Work out the finished part from the listing and answer in its coordinate system (mm). Face numbers are marked on the shaded views. A direction names the side the tool comes from. Give positions to 0.01 mm unless a question says otherwise; leave off trailing zeros. Order: outer loops, then holes, each group sorted by start corner. A loop starts at its lowest first (then second) coordinate and runs counter-clockwise, first axis right, second up. Notation, with made-up numbers: M 37,-22.75 L 82,-22.75 A14 ccw 82,3.25 Z; hole C 53,55 d11. An arc over 180 degrees is marked long. One line per item, written item: value.
from build123d import *

# Parameters (mm, degrees)
BOSS_EXTRUDE1_DEPTH = 66.04
SKETCH2_R           = 2.5
CUT_EXTRUDE1_DEPTH  = 4.175
BOSS_EXTRUDE2_DEPTH = 2.54
SKETCH4_W           = 3.175
SKETCH4_H           = 7.62
CUT_EXTRUDE2_DEPTH  = 25.4
SKETCH5_R           = 1.5
CUT_EXTRUDE3_DEPTH  = 25.4
FILLET1_R           = 3.175


with BuildPart() as part:
    # Sketch1 → Boss-Extrude1 (new body)
    with BuildSketch(Plane.XY):
        Polygon((3.175, -3.175), (15.875, -3.175), (15.875, 0), (0, 0), (0, -15.875), (3.175, -15.875), align=None)
    extrude(amount=-BOSS_EXTRUDE1_DEPTH)

    # Sketch2 → Cut-Extrude1 (cut, through all)
    with BuildSketch(Plane(origin=(3.175, 0, 0), x_dir=(0, 0, -1), z_dir=(1, 0, 0))):
        with Locations((29.95, -9.525)):
            Circle(SKETCH2_R)
        with Locations((9.95, -9.525)):
            Circle(SKETCH2_R)
    extrude(amount=-CUT_EXTRUDE1_DEPTH, mode=Mode.SUBTRACT)

    # Sketch3 → Boss-Extrude2 (add, symmetric)
    with BuildSketch(Plane.XY.offset(-19.685)):
        Polygon((3.175, -15.875), (3.175, -3.175), (15.875, -3.175), align=None)
    extrude(amount=BOSS_EXTRUDE2_DEPTH, both=True)

    # Sketch4 → Cut-Extrude2 (cut)
    with BuildSketch(Plane(origin=(0, 0, -66.04), x_dir=(-1, 0, 0), z_dir=(0, 0, -1))):
        with Locations((-1.5875, -12.065)):
            Rectangle(SKETCH4_W, SKETCH4_H)
    extrude(amount=-CUT_EXTRUDE2_DEPTH, mode=Mode.SUBTRACT)

    # Sketch5 → Cut-Extrude3 (cut)
    with BuildSketch(Plane.XZ.offset(3.175)):
        with Locations((10.375, -34.196688578)):
            Circle(SKETCH5_R)
        with Locations((10.375, -62.196688578)):
            Circle(SKETCH5_R)
    extrude(amount=-CUT_EXTRUDE3_DEPTH, mode=Mode.SUBTRACT)

    # Fillet1
    fillet1_edges = [part.edges().sort_by_distance(p)[0] for p in [
        (15.875, -1.5875, -66.04),
        (1.5875, -15.875, -40.64),
        (1.5875, -8.255, -66.04),
        (1.5875, -15.875, 0),
        (15.875, -1.5875, 0),
    ]]
    fillet(fillet1_edges, radius=FILLET1_R)


solid = part.part
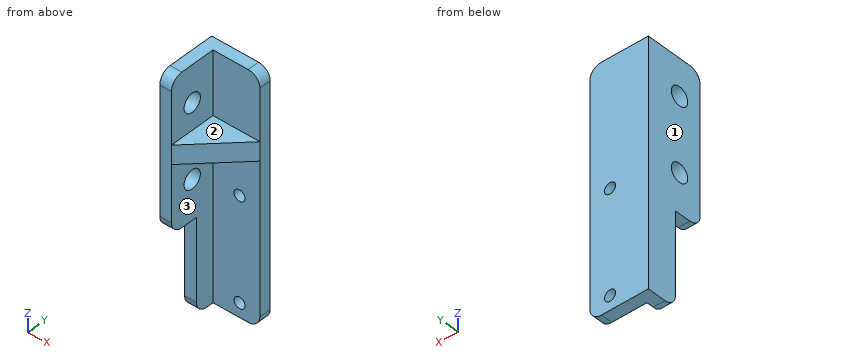
(1) Which of the six approach directions +Z, -Z, +X, -X, +Y, -Y give full straight-line access (tool end or side, diameter ignored) to the marked faces 1, 2 and 3?
Findings:
face 1: +Z, -Z, -X, +Y, -Y
face 2: +Z, +X, -Y
face 3: -Z, +X, -Y
(2) Section C-C, the plane z = -14 is taken. Give the vertices of the cut face in (x, y) (3 decimals), then the cut area to 3 significant figures.
Findings:
outline: M 0,-15.875 L 3.175,-15.875 L 3.175,-3.175 L 15.875,-3.175 L 15.875,0 L 0,0 Z
area: 90.7 mm^2
(3) Section D-D, the plane y = -10.75 is taken. Give the vertices of the cut face in (x, z) (3 decimals).
Findings:
outline: M 0,-40.64 L 3.175,-40.64 L 3.175,-32.129 L 0,-32.129 Z; M 0,-27.771 L 3.175,-27.771 L 3.175,-22.225 L 8.3,-22.225 L 8.3,-17.145 L 3.175,-17.145 L 3.175,-12.129 L 0,-12.129 Z; M 0,-7.771 L 3.175,-7.771 L 3.175,0 L 0,0 Z
(4) Section B-B, the plane x = 8.25 is taken. Give the vertices of the cut face in (y, z) (3 decimals).
Findings:
outline: M -10.8,-22.225 L -3.175,-22.225 L -3.175,-66.04 L 0,-66.04 L 0,0 L -3.175,0 L -3.175,-17.145 L -10.8,-17.145 Z
(5) Find the intervals of material crossed by probe 1 along Z at (x, y) = (11.75, -1); probe 2 along Y at (x, z) = (7.5, -41.5) (3 decimals); probe 3 along Z at (x, y) = (4.25, -6.5) (3 decimals), in increasing order. Write a range as from..to.
Findings:
probe 1: z = -66.04..-62.8, -61.6..-34.8, -33.6..0
probe 2: y = -3.175..0
probe 3: z = -22.225..-17.145
(6) Given P1, Ø2.5, axis at x = 10.38, z = -62.2, coming from the -Y side; P2, Ø6.5, axis at x = 11, y = -12.5, coming from the -Z side (3 decimals); P3, Ø1, axis at x = 11.5, y = -8, coming from the +Z side (3 decimals); P4, Ø2, axis at x = 7, z = -53.5, coming from the +Y side, each flat-ended and moving along its own axis, determine where each tip first touches the part or whether it passes through.
Findings:
P1: passes through
P2: stops at z = -22.225
P3: stops at z = -17.145
P4: stops at y = 0
(7) Section A-A, the plane z = -29.95 is taken. Give the vertices of the cut face in (x, y) (3 decimals).
Findings:
outline: M 0,-15.875 L 3.175,-15.875 L 3.175,-12.025 L 0,-12.025 Z; M 0,-7.025 L 3.175,-7.025 L 3.175,-3.175 L 15.875,-3.175 L 15.875,0 L 0,0 Z
